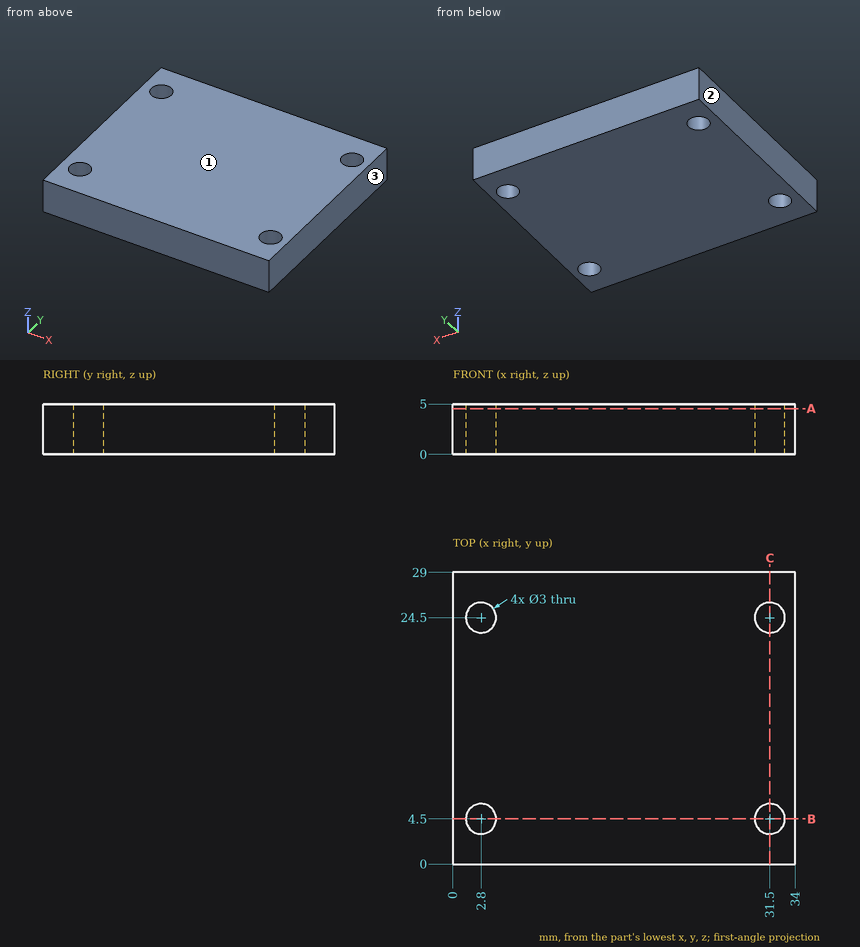
Print and shaded views of the part. All mm, measured from the part's lowest x, y and z. Give positions to 0.01 mm unless a question says otherwise; leave off trailing zeros. Loops run counter-clockwise (first coordinate to the right, second up) from the corner with the lowest first, then second, coordinate; pieces in that order, holes last. Notation, with made-up numbers: (83, 7) -> (99, 7) arc R28 cw to (99, 40) -> close; hole circle Ø10 at (64, 61.5). An arc over 180 degrees is marked (long way). Answer in a Markdown table with one row per item.
Item 1: Probe line 1 along Y through (x, z) = (31.5, 2.35); line 2 along Y through (x, z) = (32, 1.95); line 3 along X through (y, z) = (4, 1.5). List the from-to ranges inside material, lowest first. Write a range as [from, to].
Findings below:
| item | result |
|---|---|
| line 1 | y = [0, 3], [6, 23], [26, 29] |
| line 2 | y = [0, 3.09], [5.91, 23.09], [25.91, 29] |
| line 3 | x = [0, 1.39], [4.21, 30.09], [32.91, 34] |
Item 2: Slice it at A-A on z = 4.55. Write the cut outline in (x, y).
Findings below:
| item | result |
|---|---|
| outline | (0, 0) -> (34, 0) -> (34, 29) -> (0, 29) -> close; hole circle Ø3 at (2.8, 4.5); hole circle Ø3 at (2.8, 24.5); hole circle Ø3 at (31.5, 4.5); hole circle Ø3 at (31.5, 24.5) |
Item 3: Slice it at B-B on y = 4.5. Write the cut outline in (x, z).
Findings below:
| item | result |
|---|---|
| outline | (0, 0) -> (1.3, 0) -> (1.3, 5) -> (0, 5) -> close; (4.3, 0) -> (30, 0) -> (30, 5) -> (4.3, 5) -> close; (33, 0) -> (34, 0) -> (34, 5) -> (33, 5) -> close |
Item 4: Mould opens along X. For the marked faces 1, 2 and 3 say: pulls with the +X half, pulls with the -X half, needs draft (parallel to the pull), parting line crosses it, or undercut.
Findings below:
| item | result |
|---|---|
| face 1 | needs draft |
| face 2 | pulls with the -X half |
| face 3 | pulls with the +X half |
Item 5: Slice it at C-C on x = 31.5. Write the cut outline in (y, z).
Findings below:
| item | result |
|---|---|
| outline | (0, 0) -> (3, 0) -> (3, 5) -> (0, 5) -> close; (6, 0) -> (23, 0) -> (23, 5) -> (6, 5) -> close; (26, 0) -> (29, 0) -> (29, 5) -> (26, 5) -> close |
